Can you work these out from the drawing? Everything is in mm from the part's minimum corner. Give positions to 0.01 mm unless a question says otherwise; leave off trailing zeros. Write each loop counter-clockwise with the first axis right and the second up, starting at its lowest first coordinate (ties: lowest second). Pieces come first, ordered by that corner, then holes. Notation, with made-up numbers: (49.25, 22.25) - (66.25, 22.25) arc R10 cw to (66.25, 26.25) - close; hole circle Ø10 at (-16.5, 20.25). An arc over 180 degrees is marked (long way). Return JSON: item names as keys, results as strings. Group by question number.
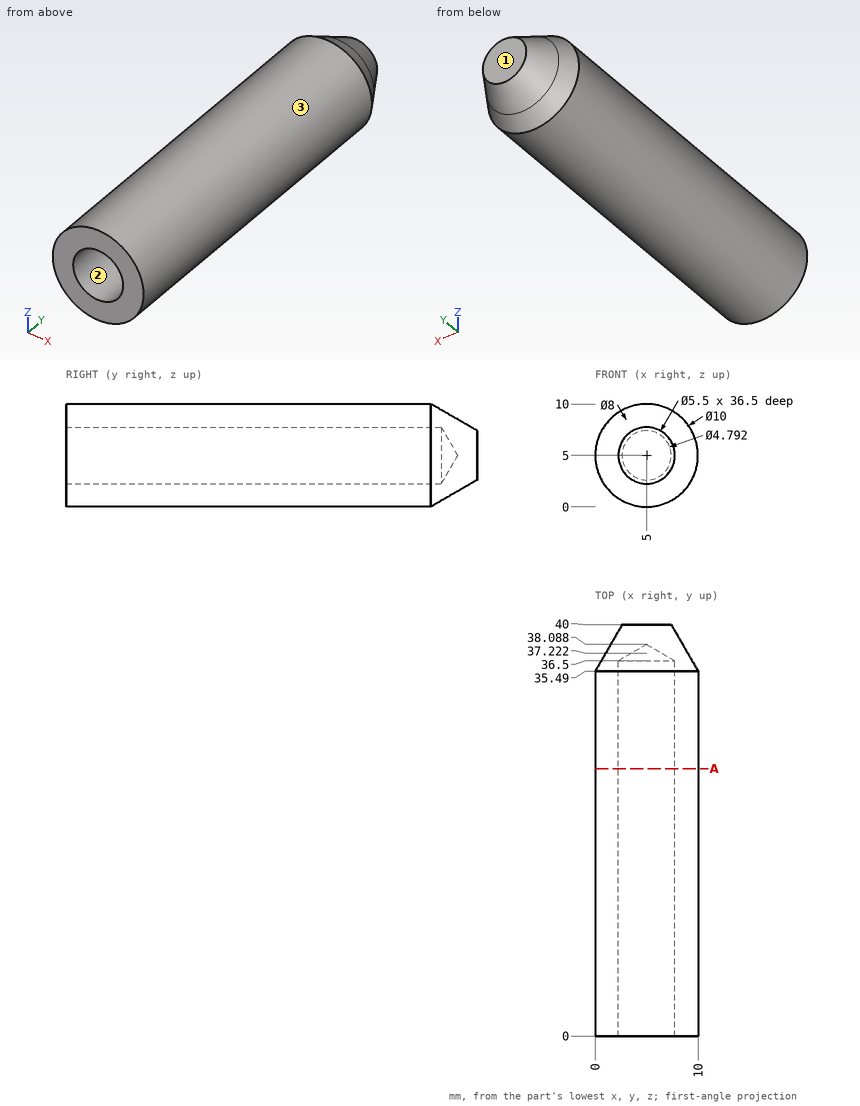
1) Will these pins go through, and if not, where does the flat tip stop? pin 1 Ø2 at (y, z) = (17, 6.5) entering from -X (1 decimal); pin 2 Ø2 at (x, y) = (3, 18) entering from +Z.
2) Imagine slicing it at A-A, the plane y = 26. Write out the boundary of the cut face in (x, z).
3) We'd pull the mould along Z, two halves only. Please class the marked faces 1, 2 and 3: pulls with the +Z half, pulls with the -Z half, needs draft (parallel to the pull), parting line crosses it, or undercut.
4) I need wall thicknesses on line 1 along Z through (x, y) = (5, 33); line 2 along Z through (x, y) = (7.5, 4) (1 decimal). Which ranges of each line are inside material? Lowest first, please.
Resolved:
{
 "1": {"pin 1": "x = 0", "pin 2": "z = 9.9"},
 "2": {"outline": "circle Ø10 at (5, 5); hole circle Ø5.5 at (5, 5)"},
 "3": {"face 1": "needs draft", "face 2": "undercut", "face 3": "parting line crosses it"},
 "4": {"line 1": "0 to 2.25, 7.75 to 10", "line 2": "0.7 to 3.9, 6.1 to 9.3"}
}
